Build history of the part. All positions in model axes, mm. A direction names the side the tool comes from. Give positions to 0.01 mm unless a question says otherwise; leave off trailing zeros. Order: outer loops, then holes, each group sorted by start corner. A loop starts at its lowest first (then second) coordinate and runs counter-clockwise, first axis right, second up. Notation, with made-up numbers: (2.5, 8.25) - (39.5, 8.25) arc R22 ccw to (39.5, 34.25) - close; hole circle Ø8 at (26, 8). An arc over 180 degrees is marked (long way). Use a Markdown table: item, result. Add a question column.
(1) Slice it at D-D (x = 0). Write the cut outline in (y, z).
(2) Mould opens along Z. For faces 3 (the face through (5, -4.4, 1.7)), 4 (the face through (0, -4, 0)), 5 (the face through (-0.54, -8.01, 8.06)), 6 (the face through (-0.54, -1.01, 8.06)) say: +Z half, -Z half, draft (parallel to the pull), parting line (faces both ways), or undercut.
(3) Slice it at C-C (z = 9). Write the cut outline in (x, y).
(4) Slice it at A-A (z = 6). Write the cut outline in (x, y).
(5) Which spindle directions (+Z, -Z, +X, -X, +Y, -Y) get a long thin tool onto all of the face, cutting with end or side? Do faces 1 (the face through (0, -2, 7)), 2 (the face through (-2, -1, 15)). Say none if no direction does.
(6) Flat gauge pin, fed straight in: pin 1 (2.5 mm diameter, centred on x = -0.5, y = -3.5, fed in from +Z). Where does the tip first touch, or does it go through?
(7) Slice it at B-B (x = -2). Write the cut outline in (y, z).
(8) Wall check: line 1 (Y direction, x = 4.25, z = 11.5); line 2 (Z direction, x = 0, y = -8); line 3 (X direction, y = -0.75, z = 12). Give the ranges that are in metal, low to high.
from build123d import *

# Parameters (mm, degrees)
F4_W      = 10
F4_H      = 15
F5_DEPTH  = 9
F6_R      = 2.5
F7_DEPTH  = 9.001
F8_R      = 4.5
F9_W      = 5
F9_H      = 13
F10_DEPTH = 10.001


with BuildPart() as f5:
    # F4 (on Front) → F5 (new body)
    with BuildSketch(Plane.XZ):
        with Locations((0, 7.5)):
            Rectangle(F4_W, F4_H)
    extrude(amount=F5_DEPTH)

    # F6 (on face) → F7 (cut, through all)
    with BuildSketch(Plane.XZ.offset(9)):
        with Locations((0, 10.5)):
            Circle(F6_R)
    extrude(amount=-F7_DEPTH, mode=Mode.SUBTRACT)

    # F8
    f8_edges = [f5.edges().sort_by_distance(p)[0] for p in [
        (5, -4.5, 15),
    ]]
    fillet(f8_edges, radius=F8_R)

    # F9 (on face) → F10 (cut, through all)
    with BuildSketch(Plane(origin=(-5, 0, 0), x_dir=(0, -1, 0), z_dir=(-1, 0, 0))):
        with Locations((4.5, 8.5)):
            Rectangle(F9_W, F9_H)
    extrude(amount=-F10_DEPTH, mode=Mode.SUBTRACT)


solid = f5.part
Solution:
| question | item | result |
|---|---|---|
| 1 | outline | (-9, 0) - (0, 0) - (0, 8) - (-2, 8) - (-2, 2) - (-7, 2) - (-7, 8) - (-9, 8) - close; (-9, 13) - (-7, 13) - (-7, 15) - (-9, 15) - close; (-2, 13) - (0, 13) - (0, 15) - (-2, 15) - close |
| 2 | face 3 | draft |
| 2 | face 4 | -Z half |
| 2 | face 5 | undercut |
| 2 | face 6 | undercut |
| 3 | outline | (-5, -9) - (-2, -9) - (-2, -7) - (-5, -7) - close; (-5, -2) - (-2, -2) - (-2, 0) - (-5, 0) - close; (2, -9) - (5, -9) - (5, -7) - (2, -7) - close; (2, -2) - (5, -2) - (5, 0) - (2, 0) - close |
| 4 | outline | (-5, -9) - (5, -9) - (5, -7) - (-5, -7) - close; (-5, -2) - (5, -2) - (5, 0) - (-5, 0) - close |
| 5 | face 1 | +Z, +X, -X |
| 5 | face 2 | +Z, +X, -X, +Y, -Y |
| 6 | pin 1 | z = 2 |
| 7 | outline | (-9, 0) - (0, 0) - (0, 9) - (-2, 9) - (-2, 2) - (-7, 2) - (-7, 9) - (-9, 9) - close; (-9, 12) - (-7, 12) - (-7, 15) - (-9, 15) - close; (-2, 12) - (0, 12) - (0, 15) - (-2, 15) - close |
| 8 | line 1 | -9 to -7, -2 to 0 |
| 8 | line 2 | 0 to 8, 13 to 15 |
| 8 | line 3 | -5 to -2, 2 to 4.74 |
